Design review of the part shown in the three views and the two pictorial views. Dimensions are in mm from the part's minimum x, y and z. A direction names the side the tool comes from. Round coordinates to 2 decimals unless told otherwise and drop trailing zeros. Loops run counter-clockwise (first coordinate to the right, second up) from the corner with the lowest first, then second, coordinate; pieces in that order, holes last. Notation, with made-up numbers: (58.25, -37.75) - (102.25, -37.75) arc R24 cw to (102.25, -7.75) - close; hole circle Ø10 at (52.25, 48). An arc over 180 degrees is marked (long way). Return JSON: item names as keys, results as strings. Group by question number.
(1) We need section C-C, the plane x = 13.25. Write out the cut boundary in (y, z).
(2) We need section A-A, the plane z = 2.75. Write out the cut boundary in (x, y).
(3) Wall thickness on L1, parallel to Y at x = 10.5, z = 0.4; L2, parallel to Y at x = 4.75, z = 2.4; L3, parallel to Z at x = 21.25, y = 1.4: over which ranges is each line inside the solid? List them lowest first. Write a range as [from, to].
(4) We need section D-D, the plane x = 20. Write out the cut boundary in (y, z), and give its area (3 significant figures).
(5) For the marked faces 1, 2 and 3, list the 3-axis set-ups (+Z, -Z, +X, -X, +Y, -Y) from which the entire face can be reached by the end or side of a thin tool; tool diameter is ignored.
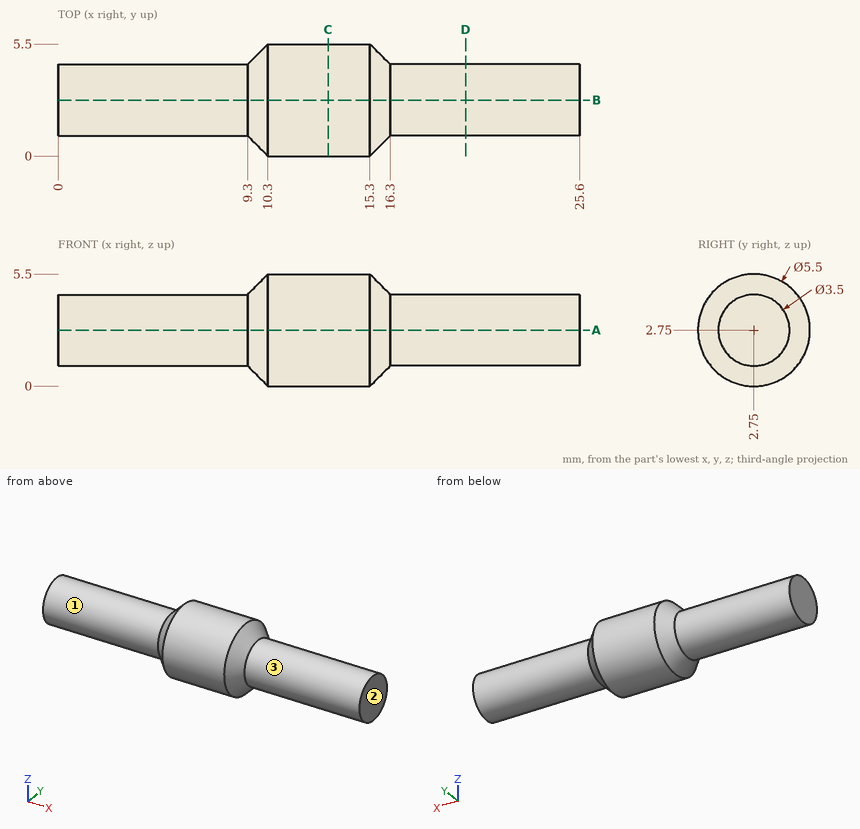
Solutions:
{
 "1": {"outline": "circle Ø5.5 at (2.75, 2.75)"},
 "2": {"outline": "(0, 1) - (9.3, 1) - (10.3, 0) - (15.3, 0) - (16.3, 1) - (25.6, 1) - (25.6, 4.5) - (16.3, 4.5) - (15.3, 5.5) - (10.3, 5.5) - (9.3, 4.5) - (0, 4.5) - close"},
 "3": {"L1": "[1.32, 4.18]", "L2": "[1.04, 4.46]", "L3": "[1.64, 3.86]"},
 "4": {"outline": "circle Ø3.5 at (2.75, 2.75)", "area": "9.62 mm^2"},
 "5": {"face 1": "-X", "face 2": "+Z, -Z, +X, +Y, -Y", "face 3": "+X"}
}
